Verification items for the finished model (mm, model axes). Face numbers are marked on the shaded views. A direction names the side the tool comes from. Round coordinates to 2 decimals unless told otherwise and drop trailing zeros. Write each loop counter-clockwise with the first axis right and the second up, starting at its lowest first coordinate (ties: lowest second). Pieces come first, ordered by that corner, then holes.
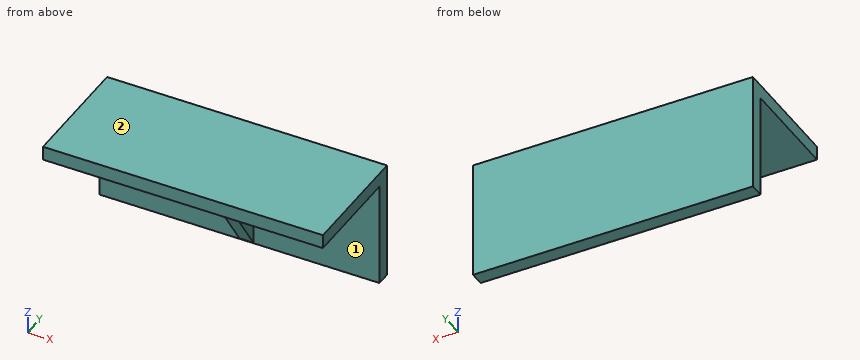
from build123d import *

# Parameters (mm, degrees)
F0_W     = 40
F0_H     = 17
F1_DEPTH = 2
F2_W     = 40
F2_H     = 2
F3_DEPTH = 15
F5_DEPTH = 2


with BuildPart() as f1:
    # F0 (on Front) → F1 (new body)
    with BuildSketch(Plane.XZ):
        Rectangle(F0_W, F0_H)
    extrude(amount=F1_DEPTH)

    # F2 (on face) → F3 (join)
    with BuildSketch(Plane.XZ.offset(2)):
        with Locations((0, 7.5)):
            Rectangle(F2_W, F2_H)
    extrude(amount=F3_DEPTH)

    # F4 (on Right) → F5 (join)
    with BuildSketch(Plane.YZ):
        Polygon((-1.942217, 6.504434), (-11.956673, 6.441844), (-1.942217, -8.517251), align=None)
    extrude(amount=F5_DEPTH)


solid = f1.part
Q1. Sectioned sample at D-D (x = 11.5). Enter the section's corners in (y, z), plus the area to 3 significant figures.
Recorded:
outline: (-17, 6.5) - (-2, 6.5) - (-2, -8.5) - (0, -8.5) - (0, 8.5) - (-17, 8.5) - close
area: 64.0 mm2
Q2. Sectioned sample at C-C (y = -10). Enter the section's corners in (x, z).
Recorded:
outline: (-20, 6.5) - (20, 6.5) - (20, 8.5) - (-20, 8.5) - close; (0, 3.52) - (2, 3.52) - (2, 6.45) - (0, 6.45) - close
Q3. Depth check by flat-ended pin: P1, Ø5, axis at x = -9.5, z = -5, coming from the -Y side; P2, Ø5, axis at y = -6.5, z = -2.5, coming from the +X side; P3, Ø5, axis at x = -0.5, z = 2.5, coming from the -Y side. Enter the tip coordinate at first touch or a pass-through.
Recorded:
P1: stops at y = -2
P2: stops at x = 2
P3: stops at y = -10.96
Q4. Sectioned sample at B-B (z = -5). Enter the section's corners in (x, y), plus the area to 3 significant figures.
Recorded:
outline: (-20, -2) - (0, -2) - (0, -4.3) - (2, -4.3) - (2, -2) - (20, -2) - (20, 0) - (-20, 0) - close
area: 84.6 mm2
Q5. Sectioned sample at A-A (y = -6.75). Enter the section's corners in (x, z), plus the area to 3 significant figures.
Recorded:
outline: (-20, 6.5) - (20, 6.5) - (20, 8.5) - (-20, 8.5) - close; (0, -1.34) - (2, -1.34) - (2, 6.47) - (0, 6.47) - close
area: 95.6 mm2
Q6. Tool access check on the marked faces 1 and 2. Record the directions out of +Z, -Z, +X, -X, +Y, -Y that give a thin tool (end or side, any length) a straight path to the whole face; none if there is none.
Recorded:
face 1: -Z, -Y
face 2: +Z, +X, -X, +Y, -Y
Q7. Material ranges on line 1 along Z through (x, y) = (15, -13.75); line 2 along Y through (x, z) = (-9, -5.5); line 3 along X through (y, z) = (-4.25, 3.5), recorded low to high.
Recorded:
line 1: z = 6.5 to 8.5
line 2: y = -2 to 0
line 3: x = 0 to 2
